```python
from build123d import *

# Parameters (mm, degrees)
SKETCH1_W           = 28
SKETCH1_H           = 8
SKETCH1_R           = 1.6
BOSS_EXTRUDE1_DEPTH = 3
SKETCH2_W           = 8
SKETCH2_H           = 8
SKETCH2_R           = 1.6
BOSS_EXTRUDE2_DEPTH = 3
FILLET1_R           = 4
FILLET2_START       = -1
FILLET2_DEPTH       = 10
FILLET2_2_DEPTH     = 8
FILLET3_R           = 0.8


with BuildPart() as part:
    # Sketch1 → Boss-Extrude1 (new body)
    with BuildSketch(Plane.XY):
        with Locations((14, 4)):
            Rectangle(SKETCH1_W, SKETCH1_H)
        with Locations((4, 4)):
            Circle(SKETCH1_R, mode=Mode.SUBTRACT)
        with Locations((24, 4)):
            Circle(SKETCH1_R, mode=Mode.SUBTRACT)
    extrude(amount=BOSS_EXTRUDE1_DEPTH)

    # Sketch2 → Boss-Extrude2 (add)
    # profile 1 of 2: a face of its own
    with BuildSketch(Plane.XY.offset(3)):
        with Locations((4, 4)):
            Rectangle(SKETCH2_W, SKETCH2_H)
        with Locations((4, 4)):
            Circle(SKETCH2_R, mode=Mode.SUBTRACT)
    # profile 2 of 2: a face of its own
    with BuildSketch(Plane.XY.offset(3)):
        with Locations((24, 4)):
            Rectangle(SKETCH2_W, SKETCH2_H)
        with Locations((24, 4)):
            Circle(SKETCH2_R, mode=Mode.SUBTRACT)
    extrude(amount=BOSS_EXTRUDE2_DEPTH)

    # Fillet1
    fillet1_edges = [part.edges().sort_by_distance(p)[0] for p in [
        (28, 8, 3),
        (28, 0, 3),
        (0, 8, 3),
        (0, 0, 3),
    ]]
    fillet(fillet1_edges, radius=FILLET1_R - 0.0001)  # a hair under: the kernel refuses the full size

    # Fillet2: read off the stored shape, not the designer's step
    # Fillet2 outline → Fillet2 (cut)
    with BuildSketch(Plane(origin=(0, 0, 0), x_dir=(1, 0, 0), z_dir=(0, 1, 0)).offset(FILLET2_START)):
        with BuildLine():
            Line((8, -6), (8, -4.5))
            ThreePointArc((8, -4.5), (7.560660172, -5.560660172), (6.5, -6))
            Line((6.5, -6), (8, -6))
        make_face()
        with BuildLine():
            ThreePointArc((21.5, -6), (20.439339828, -5.560660172), (20, -4.5))
            Line((20, -4.5), (20, -6))
            Line((20, -6), (21.5, -6))
        make_face()
    extrude(amount=FILLET2_DEPTH, mode=Mode.SUBTRACT)

    # Fillet2 2 outline → Fillet2 2 (add)
    with BuildSketch(Plane(origin=(0, 0, 0), x_dir=(1, 0, 0), z_dir=(0, 1, 0))):
        with BuildLine():
            Line((8, -3), (8, -4.5))
            ThreePointArc((8, -4.5), (8.439339828, -3.439339828), (9.5, -3))
            Line((9.5, -3), (8, -3))
        make_face()
        with BuildLine():
            Line((20, -3), (18.5, -3))
            ThreePointArc((18.5, -3), (19.560660172, -3.439339828), (20, -4.5))
            Line((20, -4.5), (20, -3))
        make_face()
    extrude(amount=FILLET2_2_DEPTH)

    # Fillet3
    fillet3_edges = [part.edges().sort_by_distance(p)[0] for p in [
        (14, 8, 0),
        (22.75005, 8, 6),
        (14, 0, 0),
        (1.171543586, 1.171543586, 0),
        (1.171543586, 6.828456414, 0),
        (26.828456414, 1.171543586, 0),
        (26.828456414, 6.828456414, 0),
        (26.828456414, 1.171543586, 6),
        (26.828456414, 6.828456414, 6),
        (5.24995, 0, 6),
        (1.171543586, 1.171543586, 6),
        (1.171543586, 6.828456414, 6),
        (5.24995, 8, 6),
        (14, 8, 3),
        (20.439339828, 8, 5.560660172),
        (7.560660172, 8, 5.560660172),
        (22.75005, 0, 6),
        (14, 0, 3),
        (20.439339828, 0, 5.560660172),
        (7.560660172, 0, 5.560660172),
        (19.560660172, 0, 3.439339828),
        (19.560660172, 8, 3.439339828),
        (8.439339828, 8, 3.439339828),
        (8.439339828, 0, 3.439339828),
    ]]
    fillet(fillet3_edges, radius=FILLET3_R)


solid = part.part
```
For this review, take the finished solid that the model builds, in its own axes (mm). A direction names the side the tool comes from. Give positions to 0.01 mm unless a question says otherwise; leave off trailing zeros. Loops run counter-clockwise (first coordinate to the right, second up) from the corner with the lowest first, then second, coordinate; pieces in that order, holes last. Notation, with made-up numbers: M -2,44 L 18,44 A14 cw 18,65 Z; hole C 59,-21.75 d5. An arc over 180 degrees is marked long. One line per item, written item: value. Start each with the question number.
Q1. Draft analysis for pull direction Y (two halves, no side actions). For faces 4 (the face through (13.86, 0.23, 0.24)), 5 (the face through (14, 8, 2)), 6 (the face through (5.48, 3.39, 2.96)), state which applies: released by +Y, released by -Y, zero draft, split by the parting line, or undercut.
Q2. Machinability: for faces 1 (the face through (14, 4, 3)), 2 (the face through (13.94, 0.23, 2.76)), 3 (the face through (14.06, 7.77, 2.76)), which of the approach directions +Z, -Z, +X, -X, +Y, -Y give a long, thin tool a straight path to every point of the face, cutting with its end or side? Answer none if there is none.
Q3. Add section A-A (x = 12.25). Give the boundary of the cut face in (y, z), and give its area (3 significant figures).
Q4. Add section B-B (y = 3.5). Count the separate pieces of the cut face and the enclosed holes in it, and give its area (3 significant figures).
Q5. Clearance check with flat-ended pins moving along their axes: pin 1 Ø1.9 at (x, y) = (12, 3) entering from +Z; pin 2 Ø1 at (x, y) = (9.5, 1) entering from +Z. State where each tip first meets the part, or that it passes through.
Q6. For L1, parallel to Y at x = 24, z = 4; L2, parallel to Z at x = 10.75, y = 7.25; L3, parallel to Y at x = 4, z = 0.35, list the stretches that pass through material, from the lowest coordinate up.
Reply:
1. face 4: released by -Y
1. face 5: released by +Y
1. face 6: undercut
2. face 1: +Z, +Y, -Y
2. face 2: +Z, -Y
2. face 3: +Z, +Y
3. outline: M 0,0.8 A0.8 ccw 0.8,0 L 7.2,0 A0.8 ccw 8,0.8 L 8,2.2 A0.8 ccw 7.2,3 L 0.8,3 A0.8 ccw 0,2.2 Z
3. area: 23.5 mm²
4. separate pieces: 3
4. enclosed holes: 0
4. area: 94.6 mm²
5. pin 1: z = 3
5. pin 2: z = 3.09
6. L1: 0 to 2.4, 5.6 to 8
6. L2: 0 to 3
6. L3: 0.14 to 2.4, 5.6 to 7.86
